CAD build for the part. Positions are in the model's coordinates, mm. A direction names the side the tool comes from. Round coordinates to 2 decimals unless told otherwise and drop trailing zeros. Order: outer loops, then holes, each group sorted by start corner. A loop starts at its lowest first (then second) coordinate and runs counter-clockwise, first axis right, second up.
```python
from build123d import *

# Parameters (mm, degrees)
SKETCH1_R           = 20
BOSS_EXTRUDE1_DEPTH = 5
CUT_EXTRUDE1_DEPTH  = 6


with BuildPart() as part:
    # Sketch1 → Boss-Extrude1 (new body)
    with BuildSketch(Plane.XY):
        with BuildLine():
            Line((-135, -120), (0, -120))
            Line((0, -120), (0, -45))
            ThreePointArc((0, -45), (-31.819805153, -31.819805153), (-45, 0))
            Line((-45, 0), (-61.846584492, 0))
            Line((-61.846584492, 0), (-200, 0))
            Line((-200, 0), (-200, -50))
            Line((-200, -50), (-175, -50))
            Line((-175, -50), (-155, -50))
            Line((-155, -50), (-155, -70))
            Line((-155, -70), (-155, -100))
            ThreePointArc((-155, -100), (-135, -80), (-115, -100))
            ThreePointArc((-115, -100), (-120.857864376, -114.142135624), (-135, -120))
        make_face()
        with BuildLine():
            ThreePointArc((-45, 0), (-44.450866059, 7.008602326), (-42.816866375, 13.846153034))
            ThreePointArc((-42.816866375, 13.846153034), (-50.079616665, 3.827848916), (-61.846584492, 0))
            Line((-61.846584492, 0), (-45, 0))
        make_face()
        with Locations((-135, -100)):
            Circle(SKETCH1_R)
        with BuildLine():
            ThreePointArc((-175, -50), (-160.857864376, -55.857864376), (-155, -70))
            Line((-155, -70), (-155, -50))
            Line((-155, -50), (-175, -50))
        make_face()
        with BuildLine():
            Line((0, -120), (41.71611649, -16.875))
            ThreePointArc((41.71611649, -16.875), (25.155764747, -37.312028891), (0, -45))
            Line((0, -45), (0, -120))
        make_face()
        with BuildLine():
            ThreePointArc((0, -45), (25.155764747, -37.312028891), (41.71611649, -16.875))
            ThreePointArc((41.71611649, -16.875), (44.171400487, -8.595776811), (45, 0))
            ThreePointArc((45, 0), (7.008602326, 44.450866059), (-42.816866375, 13.846153034))
            ThreePointArc((-42.816866375, 13.846153034), (-44.450866059, 7.008602326), (-45, 0))
            Line((-45, 0), (0, 0))
            Line((0, 0), (0, -45))
        make_face()
        with BuildLine():
            ThreePointArc((-45, 0), (-31.819805153, -31.819805153), (0, -45))
            Line((0, -45), (0, 0))
            Line((0, 0), (-45, 0))
        make_face()
    extrude(amount=BOSS_EXTRUDE1_DEPTH)

    # Sketch2 → Cut-Extrude1 (cut, through all)
    with BuildSketch(Plane.XY.offset(5)):
        with BuildLine():
            Line((-61.846584384, -15), (-185, -15))
            Line((-185, -15), (-185, -35))
            Line((-185, -35), (-175, -35))
            ThreePointArc((-175, -35), (-150.251262658, -45.251262658), (-140, -70))
            Line((-140, -70), (-140, -100))
            ThreePointArc((-140, -100), (-138.535533906, -103.535533906), (-135, -105))
            Line((-135, -105), (-10.112997937, -105))
            Line((-10.112997937, -105), (27.810744327, -11.25))
            ThreePointArc((27.810744327, -11.25), (10.246955881, 28.195742501), (-28.544577408, 9.230769231))
            ThreePointArc((-28.544577408, 9.230769231), (-41.254390195, -8.301263902), (-61.846584384, -15))
        make_face()
    extrude(amount=-CUT_EXTRUDE1_DEPTH, mode=Mode.SUBTRACT)


solid = part.part
```
1. Tool access for faces 1 (the face through (-161.014, -55.703, 2.465)), 2 (the face through (-139, -103, 3)), 3 (the face through (-130, 0, 2)): list every direction of +Z, -Z, +X, -X, +Y, -Y with a clear straight run to the whole face (end or side of a thin tool).
2. Drill centre lines: line 1 (Y direction, x = -102, z = 1.3); line 2 (Y direction, x = -188.5, z = 3.65); line 3 (Y direction, x = -56.5, z = 4.4). Where is each one in solid material? Low to high.
3. Cut at B-B, the plane x = 5. Write the cut outline in (y, z), and give its area (3 significant figures).
4. Cut at C-C, the plane y = -60.5. Write the cut outline in (x, z), and give its area (3 significant figures).
5. Cut at A-A, the plane z = 4. Write the cut outline in (x, y) (3 decimals).
6. Pin check, flat tips, straight feed: P1, Ø1.5, axis at y = -10, z = 4.5, coming from the +X side; P2, Ø2, axis at y = -92, z = 2.5, coming from the +X side; P3, Ø3, axis at x = -113.5, z = 1, coming from the +Y side. Stop position of each tip, or through.
7. Mould opens along X. For faces 4 (the face through (-155, -85, 2)), 5 (the face through (-73, -105, 3)), 6 (the face through (-69, -13, 0)) say: released by +X, released by -X, zero draft, split by the parting line, or undercut.
Outcome:
1. face 1: +Z, -Z, -X, -Y
1. face 2: +Z, -Z
1. face 3: +Z, -Z, -X, +Y
2. line 1: y = -120 to -105, -15 to 0
2. line 2: y = -50 to 0
2. line 3: y = -120 to -105, -14.59 to 0.73
3. outline: (-107.64, 0) - (-67.64, 0) - (-67.64, 5) - (-107.64, 5) - close; (29.58, 0) - (44.72, 0) - (44.72, 5) - (29.58, 5) - close
3. area: 276 mm2
4. outline: (-157.4, 0) - (-141.31, 0) - (-141.31, 5) - (-157.4, 5) - close; (7.89, 0) - (24.07, 0) - (24.07, 5) - (7.89, 5) - close
4. area: 161 mm2
5. outline: (-200, -50) - (-175, -50) arc R20 cw to (-155, -70) - (-155, -100) arc R20 ccw to (-135, -120) - (0, -120) - (41.716, -16.875) arc R45 ccw (long way) to (-42.817, 13.846) arc R20 cw to (-61.847, 0) - (-200, 0) - close; hole (-185, -35) - (-175, -35) arc R35 cw to (-140, -70) - (-140, -100) arc R5 ccw to (-135, -105) - (-10.113, -105) - (27.811, -11.25) arc R30 ccw (long way) to (-28.545, 9.231) arc R35 cw to (-61.847, -15) - (-185, -15) - close
6. P1: stops at x = 44.04
6. P2: stops at x = 11.73
6. P3: stops at y = 0
7. face 4: released by -X
7. face 5: undercut
7. face 6: zero draft
